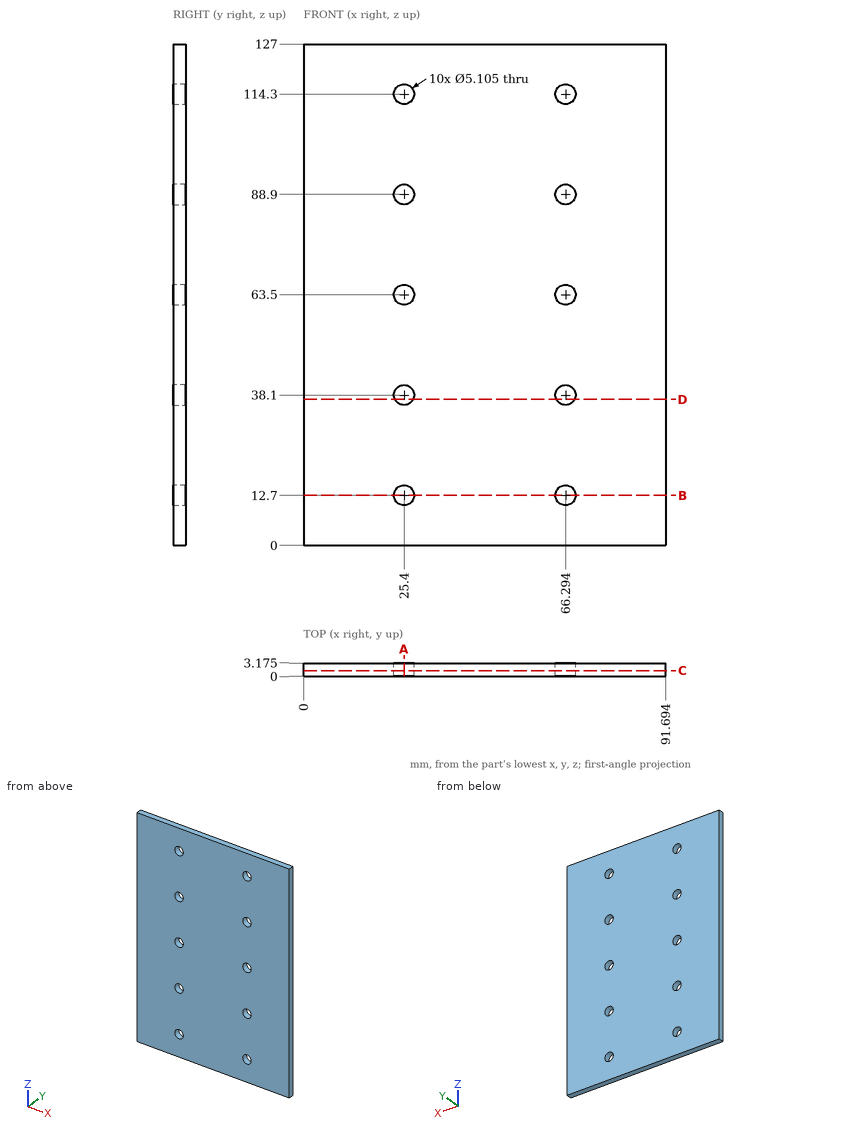
Print and shaded views of the part. All mm, measured from the part's lowest x, y and z. Coordinates: 2 decimals unless noted, no trailing zeros. Order: outer loops, then holes, each group sorted by start corner. A loop starts at its lowest first (then second) coordinate and runs counter-clockwise, first axis right, second up. Notation, with made-up numbers: (88.5, -33.75) -> (131.5, -33.75) arc R11 cw to (131.5, -23.75) -> close; hole circle Ø1 at (39, 52.25). An arc over 180 degrees is marked (long way). Use one line per item in the form item = value. Start each with the question number.
1) Band-saw the part on A-A on x = 25.4. Give the cut face in (y, z) (1 decimal).
2) Band-saw the part on D-D on z = 37. Give the cut face in (x, y) (1 decimal).
3) Band-saw the part on B-B on z = 12.7. Give the cut face in (x, y) (1 decimal), then the cut area to 3 significant figures.
4) Drop flat-ended pins along their axis: pin 1 (8 mm diameter, centred on x = 25.4, z = 63.5, fed in from +Y) (3 decimals); pin 2 (3 mm diameter, centred on x = 66.294, z = 12.7, fed in from -Y). Give the stop position or say it passes through.
5) Band-saw the part on C-C on y = 1.35. State how many separate pieces and enclosed holes the cut face has, then the cut area to 3 significant figures.
6) Drill centre lines: L1, parallel to X at y = 2, z = 12.7; L2, parallel to Z at x = 23.5, y = 1.1 (1 decimal); L3, parallel to X at y = 2.85, z = 89.5 (1 decimal). Where is each one in solid material? Low to high. Write a range as [from, to].
Entries:
q1.outline = (0, 0) -> (3.2, 0) -> (3.2, 10.1) -> (0, 10.1) -> close; (0, 15.3) -> (3.2, 15.3) -> (3.2, 35.5) -> (0, 35.5) -> close; (0, 40.7) -> (3.2, 40.7) -> (3.2, 60.9) -> (0, 60.9) -> close; (0, 66.1) -> (3.2, 66.1) -> (3.2, 86.3) -> (0, 86.3) -> close; (0, 91.5) -> (3.2, 91.5) -> (3.2, 111.7) -> (0, 111.7) -> close; (0, 116.9) -> (3.2, 116.9) -> (3.2, 127) -> (0, 127) -> close
q2.outline = (0, 0) -> (23.1, 0) -> (23.1, 3.2) -> (0, 3.2) -> close; (27.7, 0) -> (64, 0) -> (64, 3.2) -> (27.7, 3.2) -> close; (68.6, 0) -> (91.7, 0) -> (91.7, 3.2) -> (68.6, 3.2) -> close
q3.outline = (0, 0) -> (22.8, 0) -> (22.8, 3.2) -> (0, 3.2) -> close; (28, 0) -> (63.7, 0) -> (63.7, 3.2) -> (28, 3.2) -> close; (68.8, 0) -> (91.7, 0) -> (91.7, 3.2) -> (68.8, 3.2) -> close
q3.area = 259 mm2
q4.pin_1 = 3.175
q4.pin_2 = through
q5.separate_pieces = 1
q5.enclosed_holes = 10
q5.area = 11,400 mm2
q6.L1 = [0, 22.85], [27.95, 63.74], [68.85, 91.69]
q6.L2 = [0, 11], [14.4, 36.4], [39.8, 61.8], [65.2, 87.2], [90.6, 112.6], [116, 127]
q6.L3 = [0, 22.9], [27.9, 63.8], [68.8, 91.7]
